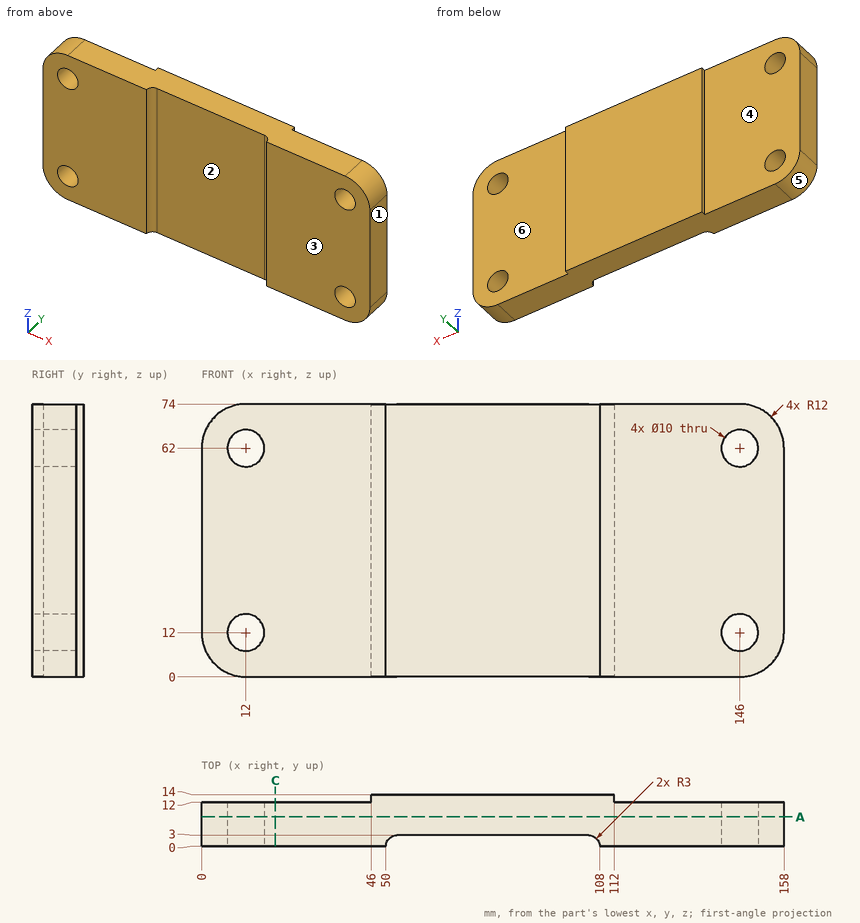
Study the drawing (mm; zero at the part's minimum x, y, z) and answer. A direction names the side the tool comes from. Coordinates: 2 decimals unless noted, no trailing zeros. Write each loop counter-clockwise with the first axis right and the second up, starting at its lowest first coordinate (ties: lowest second). Pieces come first, ordered by that corner, then holes. Notation, with made-up numbers: (0, 30.5) - (12, 30.5) arc R15 ccw to (12, 36.5) - close; hole circle Ø8 at (-38.75, -15). An arc over 180 degrees is marked (long way). One line per item, written item: value.
1) Consider line 1 along Z through (x, y) = (12, 3.5); line 2 along X through (y, z) = (4, 12.5) (3 decimals); line 3 along X through (y, z) = (2, 9). Determine where each line is inside the solid, lowest interval first. Write a range as from..to.
Geometry check:
line 1: z = 0..7, 17..57, 67..74
line 2: x = 0..7.025, 16.975..141.025, 150.975..158
line 3: x = 0.38..8, 16..50.76, 107.24..142, 150..157.62
2) A tool of negligible diameter and unlimited length cuts with its end or side. For the marked faces 4, 5 and 6, from which of +Z, -Z, +X, -X, +Y, -Y can it reach the whole face along a straight path? Write none if from no direction.
Geometry check:
face 4: +Z, -Z, -X, +Y
face 5: -Z, -X, +Y, -Y
face 6: +Z, -Z, +X, +Y
3) Each of these flat-tipped pins is pushed along its axis until it touches: pin 1 Ø15.5 at (x, z) = (75.5, 53) entering from -Y; pin 2 Ø1 at (y, z) = (13, 29) entering from -X; pin 3 Ø11.5 at (x, z) = (12, 12) entering from -Y; pin 4 Ø1 at (x, z) = (137, 29.5) entering from +Y. Where does it stop, or does it pass through?
Geometry check:
pin 1: stops at y = 3
pin 2: stops at x = 46
pin 3: stops at y = 0
pin 4: stops at y = 12
4) For a pull along X with two mould halves and no side action, classify the marked faces 1, 2 and 3 as pulls with the +X half, pulls with the -X half, needs draft (parallel to the pull), parting line crosses it, or undercut.
Geometry check:
face 1: pulls with the +X half
face 2: undercut
face 3: needs draft
5) Find section C-C (x = 20). Give the vertices of the cut face in (y, z), and give its area (3 significant figures).
Geometry check:
outline: (0, 0) - (12, 0) - (12, 74) - (0, 74) - close
area: 888 mm2
6) Find section A-A (y = 8). Give the vertices of the cut face in (x, z).
Geometry check:
outline: (0, 12) arc R12 ccw to (12, 0) - (146, 0) arc R12 ccw to (158, 12) - (158, 62) arc R12 ccw to (146, 74) - (12, 74) arc R12 ccw to (0, 62) - close; hole circle Ø10 at (12, 12); hole circle Ø10 at (12, 62); hole circle Ø10 at (146, 12); hole circle Ø10 at (146, 62)
